Check sheet for the modelled part. Datum: model origin and axes. Units: mm. A direction names the side the tool comes from. Coordinates: 2 decimals unless noted, no trailing zeros. Order: outer loops, then holes, each group sorted by start corner. A loop starts at its lowest first (then second) coordinate and runs counter-clockwise, first axis right, second up.
from build123d import *
from build123d.topology import SkipClean

# Parameters (mm, degrees)
CROQUIS1_W                 = 65
CROQUIS1_H                 = 61
CROQUIS1_W_2               = 63
CROQUIS1_H_2               = 59
SALIENTE_EXTRUIR1_DEPTH    = 30
CROQUIS1_7_R               = 3.35
CROQUIS1_7_R_2             = 2.15
SALIENTE_EXTRUIR2_DEPTH    = 20
SALIENTE_EXTRUIR2_2_DEPTH  = 20
SALIENTE_EXTRUIR4_DEPTH    = 10
CROQUIS2_W                 = 65
CROQUIS2_H                 = 61
SALIENTE_EXTRUIR5_DEPTH    = 1
CORTAR_EXTRUIR1_DEPTH      = 54.726157503
CORTAR_EXTRUIR1_DEPTH_BACK = 54.726157503
CROQUIS3_W                 = 3
CROQUIS3_H                 = 20
CORTAR_EXTRUIR2_START      = -40
CROQUIS5_R                 = 2.15
CORTAR_EXTRUIR2_DEPTH      = 40


with BuildPart() as part:
    # Croquis1 → Saliente-Extruir1 (new body)
    with BuildSketch(Plane.XY):
        Rectangle(CROQUIS1_W, CROQUIS1_H)
        Rectangle(CROQUIS1_W_2, CROQUIS1_H_2, mode=Mode.SUBTRACT)
    extrude(amount=SALIENTE_EXTRUIR1_DEPTH)

    # Croquis1_9 → Saliente-Extruir4 (add)
    with BuildSketch(Plane.XY):
        Polygon((17.5, -23.5), (31.5, -23.5), (31.5, -22.5), (18.5, -22.5), (18.5, 23.5), (31.5, 23.5), (31.5, 24.5), (17.5, 24.5), align=None)
    extrude(amount=SALIENTE_EXTRUIR4_DEPTH)



with BuildPart() as body_2:
    # Croquis1_7 → Saliente-Extruir2 (new body)
    with BuildSketch(Plane.XY):
        with Locations((-11.5, -19.5)):
            Circle(CROQUIS1_7_R)
        with Locations((-11.5, -19.5)):
            Circle(CROQUIS1_7_R_2, mode=Mode.SUBTRACT)
    extrude(amount=SALIENTE_EXTRUIR2_DEPTH)


with BuildPart() as body_3:
    # Croquis1_7 → Saliente-Extruir2 2 (new body)
    with BuildSketch(Plane.XY):
        with Locations((-11.5, 19.5)):
            Circle(CROQUIS1_7_R)
        with Locations((-11.5, 19.5)):
            Circle(CROQUIS1_7_R_2, mode=Mode.SUBTRACT)
    extrude(amount=SALIENTE_EXTRUIR2_2_DEPTH)


with BuildPart() as part_1:
    add(part.part)

    add(body_2.part)  # Saliente-Extruir5 merges body 2

    add(body_3.part)  # Saliente-Extruir5 merges body 3
    # Croquis2 → Saliente-Extruir5 (add)
    with BuildSketch(Plane(origin=(0, 0, 0), x_dir=(-1, 0, 0), z_dir=(0, 0, -1))):
        Rectangle(CROQUIS2_W, CROQUIS2_H)
    extrude(amount=SALIENTE_EXTRUIR5_DEPTH)

    # Croquis3 → Cortar-Extruir1 (cut, two sides: drawn at the far end of the back side and taken through both)
    with BuildSketch(Plane(origin=(0, 0, 0), x_dir=(0, 0, -1), z_dir=(1, 0, 0)).offset(-CORTAR_EXTRUIR1_DEPTH_BACK)):
        with Locations((-18, -1)):
            Rectangle(CROQUIS3_W, CROQUIS3_H)
    extrude(amount=CORTAR_EXTRUIR1_DEPTH + CORTAR_EXTRUIR1_DEPTH_BACK, mode=Mode.SUBTRACT)

    # Croquis5 → Cortar-Extruir2 (cut)
    with SkipClean():  # the faces are left unmerged after this step: merging them gives an invalid solid
        with BuildSketch(Plane.XY.offset(20).offset(CORTAR_EXTRUIR2_START)):
            with Locations(Location((-11.5, -19.5, 0), (0, 0, 180))):
                Circle(CROQUIS5_R)
            with Locations(Location((-11.5, 19.5, 0), (0, 0, 180))):
                Circle(CROQUIS5_R)
        extrude(amount=CORTAR_EXTRUIR2_DEPTH, mode=Mode.SUBTRACT)


solid = part_1.part
(1) Thickness scan on probe 1 along Y at (x, z) = (29.5, 3); probe 2 along X at (y, z) = (-17, 27); probe 3 along Y at (x, z) = (26, 20.5). Record the ranges inside material, lowest first.
Filled in:
probe 1: y = -30.5 to -29.5, -23.5 to -22.5, 23.5 to 24.5, 29.5 to 30.5
probe 2: x = -32.5 to -31.5, 31.5 to 32.5
probe 3: y = -30.5 to -29.5, 29.5 to 30.5
(2) Go/stop test with a flat-tipped pin: P1, Ø5, axis at x = -22.5, y = -3.5, coming from the +Z side. Record where the tip stops, or that it passes through.
Filled in:
P1: stops at z = 0
(3) Release check for a two-part mould opening along Y. For faces 1 (the flat face through (0, 0, -1)), 2 (the flat face through (0, 30.5, 15)), 3 (the flat face through (18, 8, 10)) record: +Y half, -Y half, draft (parallel to the pull), parting line (faces both ways), or undercut.
Filled in:
face 1: draft
face 2: +Y half
face 3: undercut
(4) Tool access check on faces 4 (the flat face through (-32.5, 0, 15)), 5 (the flat face through (0, 29.5, 15)). Record the directions out of +Z, -Z, +X, -X, +Y, -Y that give a thin tool (end or side, any length) a straight path to the whole face; none if there is none.
Filled in:
face 4: +Z, -Z, -X, +Y, -Y
face 5: +Z
(5) Cross-section at A-A (y = -0.5). Enter the section's corners in (x, z).
Filled in:
outline: (-32.5, -1) - (32.5, -1) - (32.5, 16.5) - (31.5, 16.5) - (31.5, 0) - (18.5, 0) - (18.5, 10) - (17.5, 10) - (17.5, 0) - (-31.5, 0) - (-31.5, 16.5) - (-32.5, 16.5) - close; (-32.5, 19.5) - (-31.5, 19.5) - (-31.5, 30) - (-32.5, 30) - close; (31.5, 19.5) - (32.5, 19.5) - (32.5, 30) - (31.5, 30) - close
(6) Cross-section at B-B (z = 25). Enter the section's corners in (x, y), and give its area (3 significant figures).
Filled in:
outline: (-32.5, -30.5) - (32.5, -30.5) - (32.5, 30.5) - (-32.5, 30.5) - close; hole (-31.5, -29.5) - (31.5, -29.5) - (31.5, 29.5) - (-31.5, 29.5) - close
area: 248 mm2
(7) Cross-section at D-D (y = -25). Enter the section's corners in (x, z).
Filled in:
outline: (-32.5, -1) - (32.5, -1) - (32.5, 30) - (31.5, 30) - (31.5, 0) - (-31.5, 0) - (-31.5, 30) - (-32.5, 30) - close
